from build123d import *

# Parameters (mm, degrees)
F0_W     = 38.1
F0_H     = 25.4
F1_DEPTH = 38.1
F3_DEPTH = 101.6
F5_DEPTH = 19.05


with BuildPart() as f1:
    # F0 (on Front) → F1 (new body)
    with BuildSketch(Plane.XZ):
        with Locations((19.05, 12.7)):
            Rectangle(F0_W, F0_H)
    extrude(amount=F1_DEPTH)

    # F2 (on face) → F3 (cut)
    with BuildSketch(Plane.XY.offset(25.4)):
        Polygon((38.1, -38.1), (38.1, -19.05), (0, -38.1), align=None)
    extrude(amount=-F3_DEPTH, mode=Mode.SUBTRACT)

    # F4 (on face) → F5 (cut)
    with BuildSketch(Plane.XY.offset(25.4)):
        Polygon((38.1, -19.05), (38.1, -6.35), (12.7, -6.35), (12.7, -31.75), align=None)
    extrude(amount=-F5_DEPTH, mode=Mode.SUBTRACT)


solid = f1.part
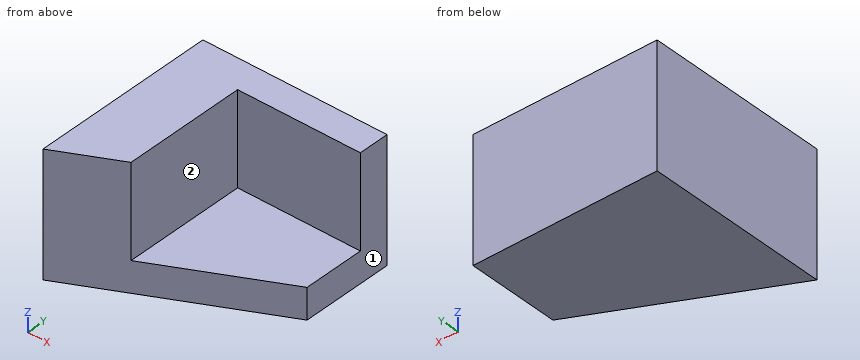
CAD build for the part. Positions are in the model's coordinates, mm. Face numbers are marked on the shaded views. A direction names the side the tool comes from. Coordinates: 2 decimals unless noted, no trailing zeros. Loops run counter-clockwise (first coordinate to the right, second up) from the corner with the lowest first, then second, coordinate; pieces in that order, holes last. Notation, with made-up numbers: (-11.5, 16.5) - (7.5, 16.5) arc R25 cw to (7.5, 41.5) - close; hole circle Ø4 at (30, 43.5). An arc over 180 degrees is marked (long way). Write item = value, one per line. Start each with the question number.
Q1. Cut at B-B, the plane z = 11.5. List the corners of the cut face in (x, y), then the cut area to 3 significant figures.
Q2. Flat gauge pins, fed straight in: pin 1 Ø8 at (x, y) = (24, -24.5) entering from +Z; pin 2 Ø6 at (y, z) = (-33, 15) entering from +X; pin 3 Ø5.5 at (x, z) = (28.5, 19.5) entering from -Y. Where does each tip first touch, or does it go through?
Q3. Cut at D-D, the plane x = 4.5. List the corners of the cut face in (y, z).
Q4. Which spindle directions (+Z, -Z, +X, -X, +Y, -Y) get a long thin tool onto all of the face, cutting with end or side? Do the marked faces 1 and 2. Say none if no direction does.
Q5. Cut at C-C, the plane y = -34.5. List the corners of the cut face in (x, z).
Q6. Drill centre lines: L1, parallel to Y at x = 24, z = 8.5; L2, parallel to X at y = -19, z = 17.25; L3, parallel to Z at x = 36.5, y = -10.5. Where is each one in solid material? Low to high.
Q7. Cut at A-A, the plane x = 23.5. List the corners of the cut face in (y, z).
Computed:
q1.outline = (0, -38.1) - (12.7, -31.75) - (12.7, -6.35) - (38.1, -6.35) - (38.1, 0) - (0, 0) - close
q1.area = 605 mm²
q2.pin_1 = 6.35
q2.pin_2 = 12.7
q2.pin_3 = -6.35
q3.outline = (-35.85, 0) - (0, 0) - (0, 25.4) - (-35.85, 25.4) - close
q4.face_1 = +Z, -Z, +X, +Y, -Y
q4.face_2 = +Z, +X, -Y
q5.outline = (0, 0) - (7.2, 0) - (7.2, 25.4) - (0, 25.4) - close
q6.L1 = -6.35 to 0
q6.L2 = 0 to 12.7
q6.L3 = 0 to 6.35
q7.outline = (-26.35, 0) - (0, 0) - (0, 25.4) - (-6.35, 25.4) - (-6.35, 6.35) - (-26.35, 6.35) - close
